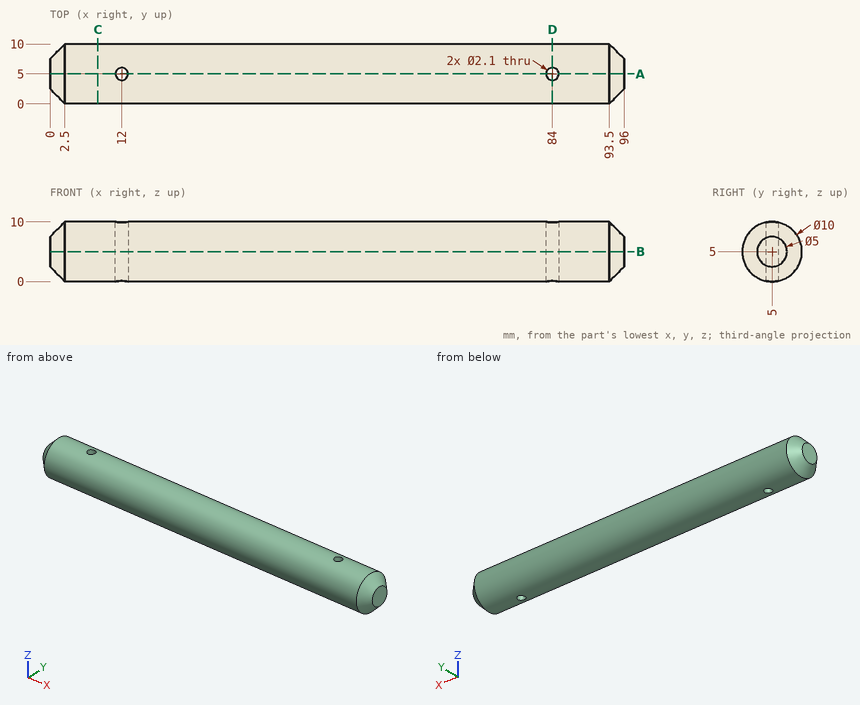
Job drawing, mm, ordinate dimensions from the low corner. One solid piece. Coordinates: 2 decimals unless noted, no trailing zeros. Order: outer loops, then holes, each group sorted by start corner. A loop starts at its lowest first (then second) coordinate and runs counter-clockwise, first axis right, second up. Notation, with made-up numbers: M 30,52.25 L 68,52.25 A15 cw 68,69.25 Z; hole C 10,89 d9. An arc over 180 degrees is marked long. Answer as CSV lines item,"result".
(1) Band-saw the part on C-C, the plane x = 8. List the corners of the cut face in (y, z).
Geometry says:
outline,"C 5,5 d10"
(2) Band-saw the part on A-A, the plane y = 5. List the corners of the cut face in (x, z).
Geometry says:
outline,"M 0,2.5 L 2.5,0 L 10.95,0 L 10.95,10 L 2.5,10 L 0,7.5 Z; M 13.05,0 L 82.95,0 L 82.95,10 L 13.05,10 Z; M 85.05,0 L 93.5,0 L 96,2.5 L 96,7.5 L 93.5,10 L 85.05,10 Z"
(3) Flat gauge pins, fed straight in: pin 1 (1 mm diameter, centred on x = 59, z = 4.5, fed in from +Y); pin 2 (5 mm diameter, centred on x = 63.5, y = 1, fed in from -Z); pin 3 (1.7 mm diameter, centred on x = 84, y = 5, fed in from -Z); pin 4 (2 mm diameter, centred on x = 67.5, z = 8, fed in from -Y). Where does each tip first touch, or does it go through?
Geometry says:
pin 1,"stops at y = 10"
pin 2,"stops at z = 0.23"
pin 3,"passes through"
pin 4,"stops at y = 0.42"
(4) Band-saw the part on D-D, the plane x = 84. List the corners of the cut face in (y, z).
Geometry says:
outline,"M 3.95,0.11 L 3.95,9.89 A5 ccw Z; M 6.05,0.11 A5 ccw 6.05,9.89 Z"
(5) Band-saw the part on B-B, the plane z = 5. List the corners of the cut face in (x, y).
Geometry says:
outline,"M 0,2.5 L 2.5,0 L 93.5,0 L 96,2.5 L 96,7.5 L 93.5,10 L 2.5,10 L 0,7.5 Z; hole C 12,5 d2.1; hole C 84,5 d2.1"
(6) Wall check: line 1 along Y through (x, z) = (84, 5.25); line 2 along X through (y, z) = (5.75, 1.5); line 3 along X through (y, z) = (4.5, 3.25). Give the ranges that are in metal, low to high.
Geometry says:
line 1,"y = 0.01 to 3.95, 6.05 to 9.99"
line 2,"x = 1.08 to 11.27, 12.73 to 83.27, 84.73 to 94.92"
line 3,"x = 0 to 11.08, 12.92 to 83.08, 84.92 to 96"
